Build history of the part. All positions in model axes, mm. A direction names the side the tool comes from. Round coordinates to 2 decimals unless told otherwise and drop trailing zeros. Loops run counter-clockwise (first coordinate to the right, second up) from the corner with the lowest first, then second, coordinate; pieces in that order, holes last. Notation, with made-up numbers: (40, 21) - (73, 21) arc R29 ccw to (73, 46) - close; hole circle Ø2 at (47.5, -16.75). An arc over 180 degrees is marked (long way). Use a Markdown table: item, result.
from build123d import *

# Parameters (mm, degrees)
BOSS_EXTRUDE1_DEPTH = 3
FILLET1_R           = 250
FILLET2_R           = 5
SKETCH2_R           = 1
CUT_EXTRUDE1_DEPTH  = 3
SKETCH3_W           = 57.60029736
SKETCH3_H           = 5
BOSS_EXTRUDE2_DEPTH = 40
FILLET3_R           = 10


with BuildPart() as part:
    # Sketch1 → Boss-Extrude1 (new body)
    with BuildSketch(Plane(origin=(0, 0, 0), x_dir=(1, 0, 0), z_dir=(0, 1, 0))):
        Polygon((-22.5, 52.5), (22.5, 52.5), (25.349290321, 7.5), (30, -30), (34.417386739, -65.618650519), (30, -65.950548022), (-30, -65.950548022), (-34.417386739, -65.618650519), (-30, -30), (-25.349290321, 7.5), align=None)
    extrude(amount=BOSS_EXTRUDE1_DEPTH)

    # Fillet1
    # the kernel refuses this fillet: 250 mm, written as the material it adds along each edge
    with BuildSketch(Plane(origin=(-25.349290321, 0, -7.5), x_dir=(-0.12307603906737652, 0, 0.9923972433493987), z_dir=(0, 1, 0))) as fillet1_piece_1:
        with BuildLine():
            CenterArc((FILLET1_R * 0.0300869468275, -FILLET1_R), FILLET1_R, 90, 3.446670391)
            Line((-FILLET1_R * 0.0300325252162, -FILLET1_R * 0.00180881135867), (0, 0))
            Line((0, 0), (FILLET1_R * 0.0300869468274, 0))
        make_face()
    extrude(amount=3)
    with BuildSketch(Plane(origin=(25.349290321, 0, -7.5), x_dir=(0.12307603906732778, 0, 0.9923972433494047), z_dir=(0, 1, 0))) as fillet1_piece_2:
        with BuildLine():
            CenterArc((FILLET1_R * 0.0300869468274, FILLET1_R), FILLET1_R, 266.553329609, 3.446670391)
            Line((-FILLET1_R * 0.0300325252162, FILLET1_R * 0.00180881135867), (0, 0))
            Line((0, 0), (FILLET1_R * 0.0300869468274, 0))
        make_face()
    extrude(amount=3)

    # Fillet2
    fillet2_edges = [part.edges().sort_by_distance(p)[0] for p in [
        (-22.5, 1.5, -52.5),
        (-34.417386739, 1.5, 65.618650519),
        (34.417386739, 1.5, 65.618650519),
        (22.5, 1.5, -52.5),
    ]]
    fillet(fillet2_edges, radius=FILLET2_R)

    # Sketch2 → Cut-Extrude1 (cut)
    with BuildSketch(Plane(origin=(0, 3, 0), x_dir=(1, 0, 0), z_dir=(0, 1, 0))):
        with Locations(Location((-14.115125166, 43.702233324, 0), (0, 0, 270))):
            Circle(SKETCH2_R)
    extrude(amount=-CUT_EXTRUDE1_DEPTH, mode=Mode.SUBTRACT)

    # Sketch3 → Boss-Extrude2 (add)
    with BuildSketch(Plane(origin=(0, 3, 0), x_dir=(1, 0, 0), z_dir=(0, 1, 0))):
        with Locations((0, -63.450548022)):
            Rectangle(SKETCH3_W, SKETCH3_H)
    extrude(amount=BOSS_EXTRUDE2_DEPTH)

    # Fillet3
    fillet3_edges = [part.edges().sort_by_distance(p)[0] for p in [
        (0, 3, 60.950548022),
    ]]
    fillet(fillet3_edges, radius=FILLET3_R)


solid = part.part
Q1. Pull direction X, two halves, no side cores. Call faces 1 (the face through (0, 21, 65.951)), 2 (the face through (25.45, 1.48, -7.62)), 3 (the face through (-23.85, 1.48, -31.18)): pulls with the +X half, pulls with the -X half, needs draft (parallel to the pull), parting line crosses it, or undercut.
Results found:
| item | result |
|---|---|
| face 1 | needs draft |
| face 2 | pulls with the +X half |
| face 3 | pulls with the -X half |
Q2. Cut at D-D, the plane x = 21. List the corners of the cut face in (y, z), plus the area to 3 significant figures.
Results found:
| item | result |
|---|---|
| outline | (0, -51.35) - (3, -51.35) - (3, 50.95) arc R10 cw to (13, 60.95) - (43, 60.95) - (43, 65.95) - (0, 65.95) - close |
| area | 573 mm2 |
Q3. Probe line 1 (Z direction, x = 2, y = 20); line 2 (Y direction, x = 3.5, z = 48.5); line 3 (Z direction, x = -15, y = 7.5). List the from-to ranges inside material, lowest first.
Results found:
| item | result |
|---|---|
| line 1 | z = 60.95 to 65.95 |
| line 2 | y = 0 to 3 |
| line 3 | z = 59.3 to 65.95 |
Q4. Drop flat-ended pins along their axis: pin 1 (3 mm diameter, centred on x = -14.12, z = -43.7, fed in from +Y); pin 2 (15 mm diameter, centred on x = -14.5, y = 26.5, fed in from -Z). Give the stop position or say it passes through.
Results found:
| item | result |
|---|---|
| pin 1 | stops at y = 3 |
| pin 2 | stops at z = 60.95 |
Q5. Which spindle directions (+Z, -Z, +X, -X, +Y, -Y) get a long thin tool onto all of the face, cutting with end or side? Do faces 4 (the face through (28.8, 23, 64)), 5 (the face through (-28.8, 23, 64)), 6 (the face through (0, 28, 60.951)). Say none if no direction does.
Results found:
| item | result |
|---|---|
| face 4 | +Z, -Z, +X, +Y |
| face 5 | +Z, -Z, -X, +Y |
| face 6 | -Z, +X, -X, +Y |
Q6. Cut at B-B, the plane y = 17. List the corners of the cut face in (x, z), plus the area to 3 significant figures.
Results found:
| item | result |
|---|---|
| outline | (-28.8, 60.95) - (28.8, 60.95) - (28.8, 65.95) - (-28.8, 65.95) - close |
| area | 288 mm2 |
Q7. Cut at A-A, the plane x = -7. List the corners of the cut face in (y, z), plus the area to 3 significant figures.
Results found:
| item | result |
|---|---|
| outline | (0, -52.5) - (3, -52.5) - (3, 50.95) arc R10 cw to (13, 60.95) - (43, 60.95) - (43, 65.95) - (0, 65.95) - close |
| area | 577 mm2 |
Q8. Cut at C-C, the plane z = 58.5. List the corners of the cut face in (x, y), plus the area to 3 significant figures.
Results found:
| item | result |
|---|---|
| outline | (-33.53, 0) - (33.53, 0) - (33.53, 3) - (28.8, 3) - (28.8, 6.44) - (-28.8, 6.44) - (-28.8, 3) - (-33.53, 3) - close |
| area | 399 mm2 |
